Source: CAD feature listing. Evaluate the final solid. Frame: model axes, mm. A direction names the side the tool comes from. Round coordinates to 2 decimals unless told otherwise and drop trailing zeros. Write each loop counter-clockwise with the first axis right and the second up, starting at its lowest first coordinate (ties: lowest second). Pieces come first, ordered by that corner, then holes. Notation, with made-up numbers: M 19,3 L 26,3 A25 ccw 26,23 Z; hole C 59,15 d11. An arc over 180 degrees is marked long. Use a Markdown table: item, result.
```python
from build123d import *

# Parameters (mm, degrees)
F0_W     = 20
F0_H     = 15
F1_DEPTH = 3
F2_R     = 2
F3_D     = 3.4
F3_DEPTH = 3
F3_TIP   = 1.0214630523


with BuildPart() as f1:
    # F0 (on Top) → F1 (new body)
    with BuildSketch(Plane.XY):
        Polygon((9.4637456983, -20.5), (20.5, -20.5), (20.5, 20.5), (-20.5, 20.5), (-20.5, -20.5), (-10.5362543017, -20.5), align=None)
        with BuildLine():
            Line((-10.2246830758, -16), (-14.7, -16))
            ThreePointArc((-14.7, -16), (-16.9192388155, -16.9192388155), (-16, -14.7))
            Line((-16, -14.7), (-16, -10.2246830758))
            ThreePointArc((-16, -10.2246830758), (-18.988, 0), (-16, 10.2246830758))
            Line((-16, 10.2246830758), (-16, 14.7))
            ThreePointArc((-16, 14.7), (-16.9192388155, 16.9192388155), (-14.7, 16))
            Line((-14.7, 16), (-10.2246830758, 16))
            ThreePointArc((-10.2246830758, 16), (0, 18.988), (10.2246830758, 16))
            Line((10.2246830758, 16), (14.7, 16))
            ThreePointArc((14.7, 16), (16, 17.3), (17.3, 16))
            ThreePointArc((17.3, 16), (16.9192388155, 15.0807611845), (16, 14.7))
            Line((16, 14.7), (16, 10.2246830758))
            ThreePointArc((16, 10.2246830758), (18.2256981211, 5.3261686042), (18.988, 0))
            ThreePointArc((18.988, 0), (18.2256981211, -5.3261686042), (16, -10.2246830758))
            Line((16, -10.2246830758), (16, -14.7))
            ThreePointArc((16, -14.7), (16.9192388155, -15.0807611845), (17.3, -16))
            ThreePointArc((17.3, -16), (16, -17.3), (14.7, -16))
            Line((14.7, -16), (10.2246830758, -16))
            ThreePointArc((10.2246830758, -16), (0, -18.988), (-10.2246830758, -16))
        make_face(mode=Mode.SUBTRACT)
        with BuildLine():
            Line((-16, 14.7), (-16, 10.2246830758))
            ThreePointArc((-16, 10.2246830758), (-13.4265435612, 13.4265435612), (-10.2246830758, 16))
            Line((-10.2246830758, 16), (-14.7, 16))
            ThreePointArc((-14.7, 16), (-15.0807611845, 15.0807611845), (-16, 14.7))
        make_face()
        with BuildLine():
            ThreePointArc((10.2246830758, 16), (13.4265435612, 13.4265435612), (16, 10.2246830758))
            Line((16, 10.2246830758), (16, 14.7))
            ThreePointArc((16, 14.7), (15.0807611845, 15.0807611845), (14.7, 16))
            Line((14.7, 16), (10.2246830758, 16))
        make_face()
        with BuildLine():
            ThreePointArc((16, -10.2246830758), (13.4265435612, -13.4265435612), (10.2246830758, -16))
            Line((10.2246830758, -16), (14.7, -16))
            ThreePointArc((14.7, -16), (15.0807611845, -15.0807611845), (16, -14.7))
            Line((16, -14.7), (16, -10.2246830758))
        make_face()
        with BuildLine():
            ThreePointArc((-16, -14.7), (-15.0807611845, -15.0807611845), (-14.7, -16))
            Line((-14.7, -16), (-10.2246830758, -16))
            ThreePointArc((-10.2246830758, -16), (-13.4265435612, -13.4265435612), (-16, -10.2246830758))
            Line((-16, -10.2246830758), (-16, -14.7))
        make_face()
        with Locations((-0.5362543017, -28)):
            Rectangle(F0_W, F0_H)
    extrude(amount=F1_DEPTH)

    # F2
    f2_edges = [f1.edges().sort_by_distance(p)[0] for p in [
        (20.5, -20.5, 1.5),
        (20.5, 20.5, 1.5),
        (-20.5, 20.5, 1.5),
        (-20.5, -20.5, 1.5),
        (-10.536254, -35.5, 1.5),
        (9.463746, -35.5, 1.5),
        (-10.536254, -20.5, 1.5),
        (9.463746, -20.5, 1.5),
    ]]
    fillet(f2_edges, radius=F2_R)

    # F3
    with Locations(Plane(origin=(0, 0, 0), x_dir=(1, 0, 0), z_dir=(0, 0, -1))):
        with Locations((-5, 28), (5, 28), (-5, 32), (5, 32)):
            Hole(F3_D / 2, depth=F3_DEPTH)
            with Locations((0, 0, -(F3_DEPTH + F3_TIP / 2))):  # 118° drill point
                Cone(0, F3_D / 2, F3_TIP, mode=Mode.SUBTRACT)


solid = f1.part
```
Q1. Mould query, pull axis Y, two halves, no side actions, for faces 3 (the flat face through (9.464, -28, 1)), 4 (the cylindrical face through (-4.63, -30.34, 1.52)), 5 (the flat face through (-1, -35.5, 1)). Classes: +Y half, -Y half, draft (parallel to the pull), parting line (faces both ways), or undercut.
Results are:
| item | result |
|---|---|
| face 3 | draft |
| face 4 | undercut |
| face 5 | -Y half |
Q2. Section C-C on y = 3.5. Return loops of the section in (x, z).
Results are:
| item | result |
|---|---|
| outline | M -20.5,0 L -18.66,0 L -18.66,3 L -20.5,3 Z; M 18.66,0 L 20.5,0 L 20.5,3 L 18.66,3 Z |
Q3. Section D-D on z = 1.2. Give the number of separate pieces and of enclosed holes in the cut face, plus the area to 3 significant figures.
Results are:
| item | result |
|---|---|
| separate pieces | 1 |
| enclosed holes | 9 |
| area | 787 mm^2 |
Q4. First-contact query: pin 1 Ø0.9 at (x, z) = (-15, 2) entering from -Y. Flat tip, straight axial feed; report the tip coordinate or a pass-through.
Results are:
| item | result |
|---|---|
| pin 1 | y = -20.5 |
Q5. Section B-B on x = 5. Return loops of the section in (y, z), plus the area to 3 significant figures.
Results are:
| item | result |
|---|---|
| outline | M -35.5,0 L -33.7,0 L -33.7,3 L -35.5,3 Z; M -30.3,0 L -29.7,0 L -29.7,3 L -30.3,3 Z; M -26.3,0 L -18.32,0 L -18.32,3 L -26.3,3 Z; M 18.32,0 L 20.5,0 L 20.5,3 L 18.32,3 Z |
| area | 37.7 mm^2 |
Q6. Reachability of faces 1 (the flat face through (-16, -20.5, 1)), 2 (the flat face through (0, -20, 0)) from +Z, -Z, +X, -X, +Y, -Y: full face, straight path, thin tool, end or side. Return the list, or none.
Results are:
| item | result |
|---|---|
| face 1 | +Z, -Z, -X, -Y |
| face 2 | -Z, +X, -X, +Y, -Y |
Q7. Line query: L1, parallel to X at y = -32, z = 2.1; L2, parallel to Y at x = -16, z = 1.1; L3, parallel to Y at x = 5, z = 2. Output: solid intervals per line, ascending.
Results are:
| item | result |
|---|---|
| L1 | -10.54 to -6.7, -3.3 to 3.3, 6.7 to 9.46 |
| L2 | -20.5 to -17.3, -14.7 to -10.22, 10.22 to 14.7, 17.3 to 20.5 |
| L3 | -35.5 to -33.7, -30.3 to -29.7, -26.3 to -18.32, 18.32 to 20.5 |
Q8. Section A-A on y = -32. Return loops of the section in (x, z).
Results are:
| item | result |
|---|---|
| outline | M -10.54,0 L -6.7,0 L -6.7,3 L -10.54,3 Z; M -3.3,0 L 3.3,0 L 3.3,3 L -3.3,3 Z; M 6.7,0 L 9.46,0 L 9.46,3 L 6.7,3 Z |
